```python
from build123d import *

# Parameters (mm, degrees)
SKETCH1_W                                        = 44.45
SKETCH1_H                                        = 60.96
BOSS_EXTRUDE1_DEPTH                              = 7.9375
CBORE_FOR_1_4_SOCKET_HEAD_CAP_SCREW1_D           = 6.7564
CBORE_FOR_1_4_SOCKET_HEAD_CAP_SCREW1_CBORE_D     = 11.1125
CBORE_FOR_1_4_SOCKET_HEAD_CAP_SCREW1_CBORE_DEPTH = 6.35
SKETCH4_W                                        = 7.62
SKETCH4_H                                        = 27.94
CUT_EXTRUDE1_DEPTH                               = 45.45
F_8_32_TAPPED_HOLE1_D                            = 3.4544


with BuildPart() as part:
    # Sketch1 → Boss-Extrude1 (new body, symmetric)
    with BuildSketch(Plane.XY):
        Rectangle(SKETCH1_W, SKETCH1_H)
    extrude(amount=BOSS_EXTRUDE1_DEPTH, both=True)

    # CBORE for 1/4 Socket Head Cap Screw1 (through all)
    with Locations(Plane.XY.offset(7.9375)):
        with Locations((-12.7, -3.81), (12.7, -3.81), (12.7, -22.86), (-12.7, -22.86)):
            CounterBoreHole(CBORE_FOR_1_4_SOCKET_HEAD_CAP_SCREW1_D / 2, CBORE_FOR_1_4_SOCKET_HEAD_CAP_SCREW1_CBORE_D / 2, CBORE_FOR_1_4_SOCKET_HEAD_CAP_SCREW1_CBORE_DEPTH)

    # Sketch4 → Cut-Extrude1 (cut, through all)
    with BuildSketch(Plane(origin=(22.225, 0, 0), x_dir=(0, 0, -1), z_dir=(1, 0, 0))):
        with Locations((4.1275, 16.51)):
            Rectangle(SKETCH4_W, SKETCH4_H)
    extrude(amount=-CUT_EXTRUDE1_DEPTH, mode=Mode.SUBTRACT)

    # #8-32 Tapped Hole1 (through all)
    with Locations(Plane.XY.offset(7.9375)):
        with Locations((0, 19.939)):
            Hole(F_8_32_TAPPED_HOLE1_D / 2)


solid = part.part
```
Build history of the part. All positions in model axes, mm. A direction names the side the tool comes from. Round coordinates to 2 decimals unless told otherwise and drop trailing zeros. Loops run counter-clockwise (first coordinate to the right, second up) from the corner with the lowest first, then second, coordinate; pieces in that order, holes last.
Item 1: Saw through at C-C (x = 0). List the corners of the cut face in (y, z).
Item 2: Drill centre lines: line 1 along X through (y, z) = (-3.5, 3.25) (3 decimals); line 2 along Y through (x, z) = (-12.7, -5.5); line 3 along X through (y, z) = (-2, -4.5) (3 decimals). Where is each one in solid material? Low to high.
Item 3: Pin check, flat tips, straight feed: P1, Ø3.5, axis at x = -12.5, y = -4, coming from the +Z side; P2, Ø1, axis at x = -7.5, y = -21, coming from the +Z side; P3, Ø1, axis at x = 3.5, z = -6.5, coming from the +Y side; P4, Ø5.5, axis at x = -14, y = -24.5, coming from the +Z side. Stop position of each tip, or through.
Item 4: Saw through at B-B (y = -22.86). List the corners of the cut face in (x, z) (1 decimal), then the cut area to 3 significant figures.
Item 5: Which spindle directions (+Z, -Z, +X, -X, +Y, -Y) get a long thin tool onto all of the face, cutting with end or side? Do faces 4 (the face through (-9, -4, 1.588)), 5 (the face through (0, 2.54, -4)), 6 (the face through (0.225, 21.652, 3.752)). Say none if no direction does.
Item 6: Saw through at A-A (z = -4). List the corners of the cut face in (x, y) (3 decimals).
Item 7: Two-plate mould, pull along X, no slides. Class faces 1 (the face through (16.3, -3.7, 1.588)), 2 (the face through (0, 16, -0.318)), 3 (the face through (22.225, -7, 2)): released by +X, released by -X, zero draft, split by the parting line, or undercut.
Item 8: Saw through at D-D (x = 12.7). List the corners of the cut face in (y, z).
Worked answers:
1. outline: (-30.48, -7.94) - (2.54, -7.94) - (2.54, -0.32) - (18.21, -0.32) - (18.21, 7.94) - (-30.48, 7.94) - close; (21.67, -0.32) - (30.48, -0.32) - (30.48, 7.94) - (21.67, 7.94) - close
2. line 1: x = -22.225 to -18.248, -7.152 to 7.152, 18.248 to 22.225
2. line 2: y = -30.48 to -26.24, -19.48 to -7.19, -0.43 to 2.54
2. line 3: x = -22.225 to -15.552, -9.848 to 9.848, 15.552 to 22.225
3. P1: passes through
3. P2: stops at z = 7.94
3. P3: stops at y = 2.54
3. P4: stops at z = 1.59
4. outline: (-22.2, -7.9) - (-16.1, -7.9) - (-16.1, 1.6) - (-18.3, 1.6) - (-18.3, 7.9) - (-22.2, 7.9) - close; (-9.3, -7.9) - (9.3, -7.9) - (9.3, 1.6) - (7.1, 1.6) - (7.1, 7.9) - (-7.1, 7.9) - (-7.1, 1.6) - (-9.3, 1.6) - close; (16.1, -7.9) - (22.2, -7.9) - (22.2, 7.9) - (18.3, 7.9) - (18.3, 1.6) - (16.1, 1.6) - close
4. area: 436 mm2
5. face 4: +Z
5. face 5: -Z, +X, -X, +Y
5. face 6: +Z, -Z
6. outline: (-22.225, -30.48) - (22.225, -30.48) - (22.225, 2.54) - (-22.225, 2.54) - close; hole circle Ø6.756 at (-12.7, -22.86); hole circle Ø6.756 at (-12.7, -3.81); hole circle Ø6.756 at (12.7, -22.86); hole circle Ø6.756 at (12.7, -3.81)
7. face 1: undercut
7. face 2: zero draft
7. face 3: released by +X
8. outline: (-30.48, -7.94) - (-26.24, -7.94) - (-26.24, 1.59) - (-28.42, 1.59) - (-28.42, 7.94) - (-30.48, 7.94) - close; (-19.48, -7.94) - (-7.19, -7.94) - (-7.19, 1.59) - (-9.37, 1.59) - (-9.37, 7.94) - (-17.3, 7.94) - (-17.3, 1.59) - (-19.48, 1.59) - close; (-0.43, -7.94) - (2.54, -7.94) - (2.54, -0.32) - (30.48, -0.32) - (30.48, 7.94) - (1.75, 7.94) - (1.75, 1.59) - (-0.43, 1.59) - close
